Verification items for the finished model (mm, model axes). Give positions to 0.01 mm unless a question says otherwise; leave off trailing zeros. Order: outer loops, then holes, each group sorted by start corner. A loop starts at its lowest first (then second) coordinate and runs counter-clockwise, first axis right, second up. Notation, with made-up numbers: (33.5, -0.75) - (75.5, -0.75) arc R21 ccw to (75.5, 14.25) - close; hole circle Ø11 at (-34, 32.25). An arc over 180 degrees is marked (long way). Answer as a JSON object with one key per item and string values.
```python
from build123d import *

# Parameters (mm, degrees)
F0_W     = 25.4
F0_H     = 88.9
F1_DEPTH = 7.9375
F2_R     = 3.96875
F3_DEPTH = 7.9375
F5_D     = 3.7973
F5_DEPTH = 12.7
F5_TIP   = 1.1408240143
F6_R     = 1.27


with BuildPart() as f1:
    # F0 (on Top) → F1 (new body)
    with BuildSketch(Plane.XY):
        with Locations((12.7, 44.45)):
            Rectangle(F0_W, F0_H)
    extrude(amount=F1_DEPTH)

    # F2 (on face) → F3 (cut, through all)
    with BuildSketch(Plane.XY.offset(7.9375)):
        with Locations((12.7, 44.45)):
            Circle(F2_R)
    extrude(amount=-F3_DEPTH, mode=Mode.SUBTRACT)

    # F5
    with Locations(Plane.YZ.offset(25.4)):
        with Locations((44.45, 3.96875)):
            Hole(F5_D / 2, depth=F5_DEPTH)
            with Locations((0, 0, -(F5_DEPTH + F5_TIP / 2))):  # 118° drill point
                Cone(0, F5_D / 2, F5_TIP, mode=Mode.SUBTRACT)

    # F6
    f6_edges = [f1.edges().sort_by_distance(p)[0] for p in [
        (25.4, 88.9, 3.96875),
        (0, 88.9, 3.96875),
        (25.4, 0, 3.96875),
        (0, 0, 3.96875),
    ]]
    fillet(f6_edges, radius=F6_R)


solid = f1.part
```
(1) Material ranges on line 1 along Y through (x, z) = (12.7, 5); line 2 along Z through (x, y) = (18.5, 44.45); line 3 along Y through (x, z) = (18.5, 3.75), recorded low to high. Write a range as [from, to].
Computed values:
{"line 1": "y = [0, 40.48], [48.42, 88.9]", "line 2": "z = [0, 2.07], [5.87, 7.94]", "line 3": "y = [0, 42.56], [46.34, 88.9]"}
(2) Section check C-C (z = 3). Record the cut outline in (x, y), then the cut area to 3 significant figures.
Computed values:
{"outline": "(0, 1.27) arc R1.27 ccw to (1.27, 0) - (24.13, 0) arc R1.27 ccw to (25.4, 1.27) - (25.4, 42.82) - (16.32, 42.82) arc R3.97 cw (long way) to (16.32, 46.08) - (25.4, 46.08) - (25.4, 87.63) arc R1.27 ccw to (24.13, 88.9) - (1.27, 88.9) arc R1.27 ccw to (0, 87.63) - close", "area": "2,180 mm²"}
(3) Release check for a two-part mould opening along Y. For faces 1 (the cylindrical face through (20.73, 42.64, 4.54)), 2 (the flat face through (13, 88.9, 4)), 3 (the flat face through (18, 45, 7.938)) record: pulls with the +Y half, pulls with the -Y half, needs draft (parallel to the pull), parting line crosses it, or undercut.
Computed values:
{"face 1": "undercut", "face 2": "pulls with the +Y half", "face 3": "needs draft"}
(4) Section check B-B (x = 12.7). Record the cut outline in (y, z).
Computed values:
{"outline": "(0, 0) - (40.48, 0) - (40.48, 7.94) - (0, 7.94) - close; (48.42, 0) - (88.9, 0) - (88.9, 7.94) - (48.42, 7.94) - close"}
(5) Section check A-A (y = 44.45). Record the cut outline in (x, z), then the cut area to 3 significant figures.
Computed values:
{"outline": "(0, 0) - (8.73, 0) - (8.73, 7.94) - (0, 7.94) - close; (16.67, 0) - (25.4, 0) - (25.4, 2.07) - (16.67, 2.07) - close; (16.67, 5.87) - (25.4, 5.87) - (25.4, 7.94) - (16.67, 7.94) - close", "area": "105 mm²"}
